```python
from build123d import *

# Parameters (mm, degrees)
F1_DEPTH = 254
F2_T     = -2.54


with BuildPart() as f1:
    # F0 (on Front) → F1 (new body)
    with BuildSketch(Plane.XZ):
        with BuildLine():
            Line((-384.231603, -0.877004), (-435.024024, 0))
            ThreePointArc((-435.024024, 0), (-350.2964, -263.195684), (-122.396574, -419.76007))
            Line((-122.396574, -419.76007), (-108.688443, -370.844568))
            ThreePointArc((-108.688443, -370.844568), (-309.554484, -232.852061), (-384.231603, -0.877004))
        make_face()
    extrude(amount=F1_DEPTH)

    # F2
    f2_openings = [f1.faces().sort_by_distance(p)[0] for p in [
        (-309.554484, -127, -232.852061),
        (-115.542508, -127, -395.302319),
        (-409.627814, -127, -0.438502),
    ]]
    offset(amount=F2_T, openings=f2_openings)


solid = f1.part
```
Could you check a few things on this model? Use its own coordinates, in mm. A direction names the side the tool comes from. Round coordinates to 2 decimals unless told otherwise and drop trailing zeros. Loops run counter-clockwise (first coordinate to the right, second up) from the corner with the lowest first, then second, coordinate; pieces in that order, holes last. Notation, with made-up numbers: (-25.75, -7) -> (19.25, -7) arc R20 cw to (19.25, 19) -> close; hole circle Ø7 at (35.25, -26). An arc over 180 degrees is marked (long way). Put each result on its own line as item: value.
Q1. Which directions (+Z, -Z, +X, -X, +Y, -Y) give clear straight access to the entire face, cutting with the end or side of a thin tool? Please do faces 1 (the flat face through (-307, -2.54, -239)), 2 (the flat face through (-321, -254, -224)).
Checks:
face 1: +Z, +X
face 2: +Z, -Z, +X, -X, -Y
Q2. I want a section at B-B on x = -176. Write out the boundary of the cut face in (y, z), and give its area (3 significant figures).
Checks:
outline: (-254, -400.82) -> (0, -400.82) -> (0, -344.82) -> (-2.54, -344.82) -> (-2.54, -398.05) -> (-251.46, -398.05) -> (-251.46, -344.82) -> (-254, -344.82) -> close
area: 973 mm2
Q3. Please list where these lines run through material, in increasing order: line 1 (Y direction, x = -310, z = -304); line 2 (X direction, y = -201, z = -63.5); line 3 (Z direction, x = -255, y = -104). Write a range as from..to.
Checks:
line 1: -254..-251.46, -2.54..0
line 2: -431.4..-428.83
line 3: -356.41..-353.29
Q4. I want a section at A-A on z = -310. Write out the boundary of the cut face in (x, y).
Checks:
outline: (-309.87, -254) -> (-232.45, -254) -> (-232.45, -251.46) -> (-306.27, -251.46) -> (-306.27, -2.54) -> (-232.45, -2.54) -> (-232.45, 0) -> (-309.87, 0) -> close
Q5. For pin 1 Ø1 at (y, z) = (-73, -167.5) entering from -X; pin 2 Ø12 at (x, y) = (-387.5, -217.5) entering from -Z; pin 3 Ø10 at (y, z) = (-113.5, -146) entering from -X, each with a flat end and sliding along its axis, tell me the tip position at first contact or that it passes through.
Checks:
pin 1: x = -404.23
pin 2: z = -214.82
pin 3: x = -413.71
Q6. I want a section at C-C on y = -129. Write out the boundary of the cut face in (x, z).
Checks:
outline: (-435.02, 0) arc R428.25 ccw to (-122.4, -419.76) -> (-121.71, -417.31) arc R425.71 cw to (-432.48, -0.04) -> close
Q7. Thinking about a two-plate mould opening in Y: for faces 3 (the flat face through (-321, 0, -224)), 4 (the flat face through (-307, -251.46, -239)), 5 (the cylindrical face through (-352.64, -125.22, -260.02)), which applies, pulls with the +Y half, pulls with the -Y half, needs draft (parallel to the pull), parting line crosses it, or undercut?
Checks:
face 3: pulls with the +Y half
face 4: undercut
face 5: needs draft
